Work out the finished part from the listing and answer in its coordinate system (mm). Face numbers are marked on the shaded views. Coordinates: 2 decimals unless noted, no trailing zeros. Write each loop counter-clockwise with the first axis right and the second up, starting at its lowest first coordinate (ties: lowest second). Pieces come first, ordered by that corner, then holes. Notation, with made-up numbers: (80.25, 84) - (106.25, 84) arc R19 cw to (106.25, 88) - close; hole circle Ø5 at (-27, 51). An arc over 180 degrees is marked (long way). Use one line per item in the form item = value. Start each with the question number.
Item 1: Given pin 1 (3 mm diameter, centred on x = 4.5, y = -6.5, fed in from -Z), flat-ended and moving along its own axis, determine where the tip first touches the part or whether it passes through.
Item 2: A cutting plane is placed at D-D (y = -6). Write down the section's boundary in (x, z), then the cut area to 3 significant figures.
Item 3: Determine the mould class of the marked faces 1, 2, 3 and 4 for opening direction Y: released by +Y, released by -Y, zero draft, split by the parting line, or undercut.
Item 4: Consider probe 1 along Y at (x, z) = (-3.75, 1.5); probe 2 along Y at (x, z) = (4.5, 0.6); probe 3 along Y at (x, z) = (-4.5, -1.75). Determine where each line is inside the solid, lowest interval first.
Item 5: A cutting plane is placed at A-A (z = 0). Write down the section's boundary in (x, y).
Item 6: A cutting plane is placed at B-B (x = 5.75). Write down the section's boundary in (y, z), then the cut area to 3 significant figures.
Item 7: A cutting plane is placed at C-C (z = 2). Write down the section's boundary in (x, y).
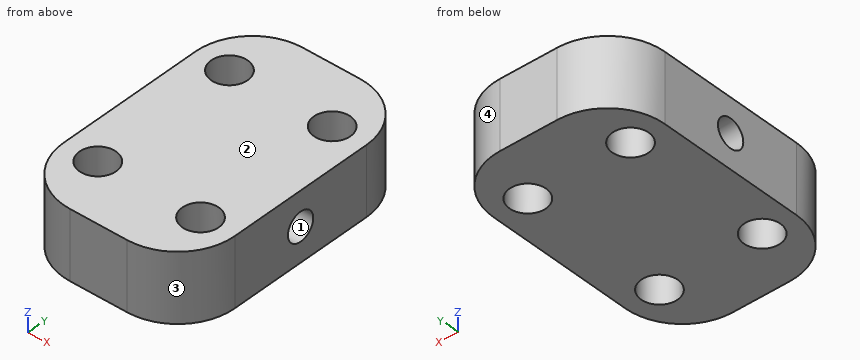
from build123d import *

# Parameters (mm, degrees)
SKETCH_1_W         = 15
SKETCH_1_H         = 23
EXTRUDE_1_DEPTH    = 3
FILLET_1_R         = 5
HOLE_WIZARD_M3_1_D = 3.2
M3X0_5_1_D         = 2.5


with BuildPart() as part:
    # ｽｹｯﾁ1 → ﾎﾞｽ - 押し出し1 (new, symmetric)
    with BuildSketch(Plane.XY):
        Rectangle(SKETCH_1_W, SKETCH_1_H)
    extrude(amount=EXTRUDE_1_DEPTH, both=True)

    # ﾌｨﾚｯﾄ1
    fillet_1_edges = [part.edges().sort_by_distance(p)[0] for p in [
        (7.5, -11.5, 0),
        (-7.5, -11.5, 0),
        (-7.5, 11.5, 0),
        (7.5, 11.5, 0),
    ]]
    fillet(fillet_1_edges, radius=FILLET_1_R)

    # M3 すきま穴1 (through all)
    with Locations(Plane(origin=(-4.5, 6.5, 3), x_dir=(1, 0, 0), z_dir=(0, 0, 1))):
        with Locations((0, 0), (9, 0), (9, -13), (0, -13)):
            Hole(HOLE_WIZARD_M3_1_D / 2)

    # M3x0.5 ねじ穴1 (through all)
    with Locations(Plane.YZ.offset(7.5)):
        with Locations((0, 0)):
            Hole(M3X0_5_1_D / 2)


solid = part.part
Answer:
q1.pin_1 = through
q2.outline = (-7.5, -3) - (-6.02, -3) - (-6.02, 3) - (-7.5, 3) - close; (-2.98, -3) - (2.98, -3) - (2.98, 3) - (-2.98, 3) - close; (6.02, -3) - (7.5, -3) - (7.5, 3) - (6.02, 3) - close
q2.area = 53.5 mm²
q3.face_1 = undercut
q3.face_2 = zero draft
q3.face_3 = released by -Y
q3.face_4 = released by +Y
q4.probe_1 = -11.34 to -7.91, -5.09 to 5.09, 7.91 to 11.34
q4.probe_2 = -11.08 to -8.1, -4.9 to -1.1, 1.1 to 4.9, 8.1 to 11.08
q4.probe_3 = -11.08 to -8.1, -4.9 to 4.9, 8.1 to 11.08
q5.outline = (-7.5, -6.5) arc R5 ccw to (-2.5, -11.5) - (2.5, -11.5) arc R5 ccw to (7.5, -6.5) - (7.5, -1.25) - (-7.5, -1.25) - close; (-7.5, 1.25) - (7.5, 1.25) - (7.5, 6.5) arc R5 ccw to (2.5, 11.5) - (-2.5, 11.5) arc R5 ccw to (-7.5, 6.5) - close; hole circle Ø3.2 at (-4.5, -6.5); hole circle Ø3.2 at (-4.5, 6.5); hole circle Ø3.2 at (4.5, -6.5); hole circle Ø3.2 at (4.5, 6.5)
q6.outline = (-10.3, -3) - (-7.5, -3) - (-7.5, 3) - (-10.3, 3) - close; (-5.5, -3) - (5.5, -3) - (5.5, 3) - (-5.5, 3) - close; (7.5, -3) - (10.3, -3) - (10.3, 3) - (7.5, 3) - close; hole circle Ø2.5 at (0, 0)
q6.area = 94.7 mm²
q7.outline = (-7.5, -6.5) arc R5 ccw to (-2.5, -11.5) - (2.5, -11.5) arc R5 ccw to (7.5, -6.5) - (7.5, 6.5) arc R5 ccw to (2.5, 11.5) - (-2.5, 11.5) arc R5 ccw to (-7.5, 6.5) - close; hole circle Ø3.2 at (-4.5, -6.5); hole circle Ø3.2 at (-4.5, 6.5); hole circle Ø3.2 at (4.5, -6.5); hole circle Ø3.2 at (4.5, 6.5)
